```python
from build123d import *

# Parameters (mm, degrees)
BOSS_EXTRUDE1_DEPTH = 12.7
SKETCH2_R           = 2.675
CUT_EXTRUDE1_DEPTH  = 16.24
SKETCH3_W           = 7.62
SKETCH3_H           = 3.81
CUT_EXTRUDE2_DEPTH  = 99.9300001


with BuildPart() as part:
    # Sketch1 → Boss-Extrude1 (new body)
    with BuildSketch(Plane.XY):
        with BuildLine():
            Line((-49.465, 0), (49.465, 0))
            Line((49.465, 0), (49.465, -15.24))
            ThreePointArc((49.465, -15.24), (0, -10.115578278), (-49.465, -15.24))
            Line((-49.465, -15.24), (-49.465, 0))
        make_face()
    extrude(amount=BOSS_EXTRUDE1_DEPTH)

    # Sketch2 → Cut-Extrude1 (cut, through all)
    with BuildSketch(Plane(origin=(0, 0, 0), x_dir=(1, 0, 0), z_dir=(0, 1, 0))):
        with Locations((-42.465, -6.35)):
            Circle(SKETCH2_R)
        with Locations((42.465, -6.35)):
            Circle(SKETCH2_R)
    extrude(amount=-CUT_EXTRUDE1_DEPTH, mode=Mode.SUBTRACT)

    # Sketch3 → Cut-Extrude2 (cut, through all)
    with BuildSketch(Plane(origin=(49.465, 0, 0), x_dir=(0, 0, -1), z_dir=(1, 0, 0))):
        with Locations((-6.35, -13.335)):
            Rectangle(SKETCH3_W, SKETCH3_H)
    extrude(amount=-CUT_EXTRUDE2_DEPTH, mode=Mode.SUBTRACT)


solid = part.part
```
Check sheet for the modelled part. Datum: model origin and axes. Units: mm. A direction names the side the tool comes from. Round coordinates to 2 decimals unless told otherwise and drop trailing zeros. Order: outer loops, then holes, each group sorted by start corner. A loop starts at its lowest first (then second) coordinate and runs counter-clockwise, first axis right, second up. Notation, with made-up numbers: M -26,-14.75 L 15,-14.75 A18 ccw 15,7.25 Z; hole C 42.25,21.5 d7. An arc over 180 degrees is marked long. Answer in a Markdown table with one row per item.
(1) Gauge pin test, flat ends, axial feed: pin 1 (2 mm diameter, centred on y = -12.5, z = 7, fed in from -X); pin 2 (4 mm diameter, centred on x = -17.5, z = 10, fed in from -Y). Record the tip position at first contact, or that the pin passes through.
Findings:
| item | result |
|---|---|
| pin 1 | passes through |
| pin 2 | stops at y = -10.9 |
(2) Draft check along X on faces 3 (the flat face through (43, -13, 10.16)), 4 (the flat face through (-49.465, -8, 6)), 5 (the cylindrical face through (0.697, -10.117, 6.261)). Enter one of: +X half, -X half, draft (parallel to the pull), parting line (faces both ways), or undercut.
Findings:
| item | result |
|---|---|
| face 3 | draft |
| face 4 | -X half |
| face 5 | undercut |
(3) Material ranges on line 1 along X through (y, z) = (-7.5, 6.35) (3 decimals); line 2 along Y through (x, z) = (37, 9); line 3 along X through (y, z) = (-10, 5) (3 decimals), recorded low to high. Write a range as from..to.
Findings:
| item | result |
|---|---|
| line 1 | x = -49.465..-45.14, -39.79..39.79, 45.14..49.465 |
| line 2 | y = -11.43..0 |
| line 3 | x = -49.465..-44.774, -40.156..40.156, 44.774..49.465 |
(4) Section check C-C on x = -42. Record the boundary of the cut face in (y, z), plus the area to 3 significant figures.
Findings:
| item | result |
|---|---|
| outline | M -13.8,0 L 0,0 L 0,3.72 L -11.43,3.72 L -11.43,2.54 L -13.8,2.54 Z; M -13.8,10.16 L -11.43,10.16 L -11.43,8.98 L 0,8.98 L 0,12.7 L -13.8,12.7 Z |
| area | 97.0 mm^2 |
(5) Section check B-B on y = -9. Record the boundary of the cut face in (x, z) (3 decimals), plus the area to 3 significant figures.
Findings:
| item | result |
|---|---|
| outline | M -49.465,0 L 49.465,0 L 49.465,12.7 L -49.465,12.7 Z; hole C -42.465,6.35 d5.35; hole C 42.465,6.35 d5.35 |
| area | 1,210 mm^2 |
(6) Set-up check for faces 1 (the flat face through (-1, 0, 6)), 2 (the flat face through (-37, -11.43, 6)): record each of +Z, -Z, +X, -X, +Y, -Y from which the full face is reachable in a straight line by a thin tool's end or side.
Findings:
| item | result |
|---|---|
| face 1 | +Z, -Z, +X, -X, +Y |
| face 2 | +X, -X, -Y |
(7) Section check D-D on y = -12.75. Record the boundary of the cut face in (x, z) (3 decimals), plus the area to 3 significant figures.
Findings:
| item | result |
|---|---|
| outline | M -49.465,0 L -35.559,0 L -35.559,2.54 L -49.465,2.54 Z; M -49.465,10.16 L -35.559,10.16 L -35.559,12.7 L -49.465,12.7 Z; M 35.559,0 L 49.465,0 L 49.465,2.54 L 35.559,2.54 Z; M 35.559,10.16 L 49.465,10.16 L 49.465,12.7 L 35.559,12.7 Z |
| area | 141 mm^2 |
(8) Section check A-A on z = 6.35. Record the boundary of the cut face in (x, y) (3 decimals), plus the area to 3 significant figures.
Findings:
| item | result |
|---|---|
| outline | M -49.465,-11.43 L -45.14,-11.43 L -45.14,0 L -49.465,0 Z; M -39.79,-11.43 L -25.152,-11.43 A241.3 cw 25.152,-11.43 L 39.79,-11.43 L 39.79,0 L -39.79,0 Z; M 45.14,-11.43 L 49.465,-11.43 L 49.465,0 L 45.14,0 Z |
| area | 964 mm^2 |
